Here's how the part is built. I have some questions about the finished solid (model axes, mm). A direction names the side the tool comes from. Round coordinates to 2 decimals unless told otherwise and drop trailing zeros. Loops run counter-clockwise (first coordinate to the right, second up) from the corner with the lowest first, then second, coordinate; pieces in that order, holes last. Notation, with made-up numbers: M 66,66 L 122,66 A6 ccw 122,73 Z; hole C 12,84.5 d1. An arc over 180 degrees is marked long. Put each result on its own line as item: value. Start each with the question number.
```python
from build123d import *

# Parameters (mm, degrees)
CROQUIS2_R              = 4
SALIENTE_EXTRUIR1_DEPTH = 70
CROQUIS3_W              = 3
CROQUIS3_H              = 7.416198488
SALIENTE_EXTRUIR2_DEPTH = 10
CROQUIS4_W              = 3
CROQUIS4_H              = 7.416198488
SALIENTE_EXTRUIR3_DEPTH = 10
CROQUIS5_R              = 1.5
CORTAR_EXTRUIR1_DEPTH   = 81.288542146
REDONDEO1_R             = 4


with BuildPart() as part:
    # Croquis2 → Saliente-Extruir1 (new body)
    with BuildSketch(Plane.XY):
        Circle(CROQUIS2_R)
    extrude(amount=SALIENTE_EXTRUIR1_DEPTH)

    # Croquis3 → Saliente-Extruir2 (add)
    with BuildSketch(Plane.XY.offset(70)):
        Rectangle(CROQUIS3_W, CROQUIS3_H)
    extrude(amount=SALIENTE_EXTRUIR2_DEPTH)

    # Croquis4 → Saliente-Extruir3 (add)
    with BuildSketch(Plane(origin=(0, 0, 0), x_dir=(-1, 0, 0), z_dir=(0, 0, -1))):
        Rectangle(CROQUIS4_W, CROQUIS4_H)
    extrude(amount=SALIENTE_EXTRUIR3_DEPTH)

    # Croquis5 → Cortar-Extruir1 (cut, through all)
    with BuildSketch(Plane(origin=(1.5, 0, 0), x_dir=(0, 0, -1), z_dir=(1, 0, 0))):
        with Locations((-75, 0)):
            Circle(CROQUIS5_R)
        with Locations((5, 0)):
            Circle(CROQUIS5_R)
    extrude(amount=-CORTAR_EXTRUIR1_DEPTH, mode=Mode.SUBTRACT)

    # Redondeo1
    # the kernel refuses this fillet: 4 mm, written as the material it takes off along each edge
    with BuildSketch(Plane(origin=(-11.5, -3.708099244, -10), x_dir=(0, 0, 1), z_dir=(1, 0, 0)), Plane(origin=(11.5, 3.708099244, -10), x_dir=(0, 0, 1), z_dir=(-1, 0, 0))) as redondeo1_piece_1:
        with BuildLine():
            CenterArc((REDONDEO1_R, -REDONDEO1_R), REDONDEO1_R, 90, 90)
            Line((0, -REDONDEO1_R), (0, 0))
            Line((0, 0), (REDONDEO1_R, 0))
        make_face()
    extrude(amount=23, mode=Mode.SUBTRACT)
    with BuildSketch(Plane(origin=(-11.5, -3.708099244, 80), x_dir=(0, 0, -1), z_dir=(1, 0, 0)), Plane(origin=(11.5, 3.708099244, 80), x_dir=(0, 0, -1), z_dir=(-1, 0, 0))) as redondeo1_piece_2:
        with BuildLine():
            CenterArc((REDONDEO1_R, REDONDEO1_R), REDONDEO1_R, 180, 90)
            Line((0, REDONDEO1_R), (0, 0))
            Line((0, 0), (REDONDEO1_R, 0))
        make_face()
    extrude(amount=23, mode=Mode.SUBTRACT)


solid = part.part
```
1) Suppose I cut it at A-A (z = 75). Write out the boundary of the cut face in (x, y).
2) If I drill on probe 1 along Y at (x, z) = (1.25, -5); probe 2 along Z at (x, y) = (-0.25, 1); probe 3 along X at (y, z) = (-3, -5.5), over which ranges is the centre line in solid material (lowest first)? Write a range as from..to.
3) Suppose I cut it at B-B (x = 0). Write out the boundary of the cut face in (y, z), plus the area to 3 significant figures.
4) Suppose I cut it at D-D (z = -2). Write out the boundary of the cut face in (x, y).
5) If we mould it in two halves opening along Z, with no side actions, what happens to faces 1 (the face through (0.021, 2.609, 78.754)), 2 (the face through (2, 0, 0)), 3 (the face through (0.021, -0.575, -6.386)), 4 (the face through (-1.5, 2, 75))? For each: pulls with the +Z half, pulls with the -Z half, needs draft (parallel to the pull), parting line crosses it, or undercut.
6) Suppose I cut it at C-C (y = 2.5). Write out the boundary of the cut face in (x, z).
7) On a 3-axis mill with a long thin cutter (end or side, diameter ignored), from which of +Z, -Z, +X, -X, +Y, -Y can I reach the whole of each face in a straight line? I mean faces 5 (the face through (-1.5, 2, -5)), 6 (the face through (1.5, 2, -5)), 7 (the face through (-2, 0, 70)), 8 (the face through (0, 3.708, 73)), 9 (the face through (0, -3.708, 73)). Say none if no direction works.
8) I'm going to push flat-ended pins straight in: P1, Ø3.5, axis at y = -1.5, z = 74, coming from the +X side; P2, Ø0.9, axis at x = 0.5, z = 72, coming from the +Y side; P3, Ø1.5, axis at x = 1.5, y = -3, coming from the -Z side. Where does each tip first touch, or does it pass through?
Results are:
1. outline: M -1.5,-3.71 L 1.5,-3.71 L 1.5,-1.5 L -1.5,-1.5 Z; M -1.5,1.5 L 1.5,1.5 L 1.5,3.71 L -1.5,3.71 Z
2. probe 1: -3.71..-1.5, 1.5..3.71
2. probe 2: -9.79..-6.12, -3.88..73.88, 76.12..79.79
2. probe 3: -1.5..1.5
3. outline: M -4,0 L -3.71,0 L -3.71,-6 A4 ccw 0,-9.99 A4 ccw 3.71,-6 L 3.71,0 L 4,0 L 4,70 L 3.71,70 L 3.71,76 A4 ccw 0,79.99 A4 ccw -3.71,76 L -3.71,70 L -4,70 Z; hole C 0,-5 d3; hole C 0,75 d3
3. area: 680 mm²
4. outline: M -1.5,-3.71 L 1.5,-3.71 L 1.5,3.71 L -1.5,3.71 Z
5. face 1: pulls with the +Z half
5. face 2: pulls with the -Z half
5. face 3: undercut
5. face 4: needs draft
6. outline: M -3.12,0 L -1.5,0 L -1.5,-8.86 L 1.5,-8.86 L 1.5,0 L 3.12,0 L 3.12,70 L 1.5,70 L 1.5,78.86 L -1.5,78.86 L -1.5,70 L -3.12,70 Z
7. face 5: -Z, -X, +Y, -Y
7. face 6: -Z, +X, +Y, -Y
7. face 7: +Z, -X, +Y, -Y
7. face 8: +Z, +X, -X, +Y
7. face 9: +Z, +X, -X, -Y
8. P1: x = 1.5
8. P2: y = 3.71
8. P3: z = -9.09
